For this review, take the finished solid that the model builds, in its own axes (mm). A direction names the side the tool comes from. Round coordinates to 2 decimals unless told otherwise and drop trailing zeros. Write each loop counter-clockwise with the first axis right and the second up, starting at its lowest first coordinate (ties: lowest second). Pieces come first, ordered by that corner, then holes.
from build123d import *

# Parameters (mm, degrees)
SKETCH1_W           = 285.8
SKETCH1_H           = 25.4
BOSS_EXTRUDE1_DEPTH = 25.4
SKETCH2_W           = 23
SKETCH2_H           = 23
CUT_EXTRUDE1_DEPTH  = 450
CUT_EXTRUDE2_DEPTH  = 25.4


with BuildPart() as part:
    # Sketch1 → Boss-Extrude1 (new body)
    with BuildSketch(Plane(origin=(0, 0, 0), x_dir=(1, 0, 0), z_dir=(0, 1, 0))):
        with Locations((142.9, 12.7)):
            Rectangle(SKETCH1_W, SKETCH1_H)
    extrude(amount=BOSS_EXTRUDE1_DEPTH)

    # Sketch2 → Cut-Extrude1 (cut)
    with BuildSketch(Plane(origin=(285.8, 0, 0), x_dir=(0, 0, -1), z_dir=(1, 0, 0))):
        with Locations((12.7, 12.7)):
            Rectangle(SKETCH2_W, SKETCH2_H)
    extrude(amount=-CUT_EXTRUDE1_DEPTH, mode=Mode.SUBTRACT)

    # Sketch3 → Cut-Extrude2 (cut)
    with BuildSketch(Plane(origin=(0, 25.4, 0), x_dir=(1, 0, 0), z_dir=(0, 1, 0))):
        Polygon((0, 0), (25.4, 25.4), (0, 25.4), align=None)
        Polygon((285.8, 0), (260.4, 25.4), (285.8, 25.4), align=None)
    extrude(amount=-CUT_EXTRUDE2_DEPTH, mode=Mode.SUBTRACT)


solid = part.part
(1) We need section C-C, the plane y = 11. Give the boundary of the cut face in (x, z).
Geometry check:
outline: (0, 0) - (1.2, -1.2) - (284.6, -1.2) - (285.8, 0) - close; (24.2, -24.2) - (25.4, -25.4) - (260.4, -25.4) - (261.6, -24.2) - close
(2) We need section A-A, the plane z = -14.75. Give the boundary of the cut face in (x, y).
Geometry check:
outline: (14.75, 0) - (271.05, 0) - (271.05, 1.2) - (14.75, 1.2) - close; (14.75, 24.2) - (271.05, 24.2) - (271.05, 25.4) - (14.75, 25.4) - close
(3) For faces 5 (the face through (145, 13, -1.2)), 6 (the face through (274.1, 0.5, -11.7)), list the 3-axis set-ups (+Z, -Z, +X, -X, +Y, -Y) from which the entire face can be reached by the end or side of a thin tool; tool diameter is ignored.
Geometry check:
face 5: +X, -X
face 6: -Z, +X, +Y, -Y
(4) We need section B-B, the plane x = 202. Give the boundary of the cut face in (y, z), and give its area (3 significant figures).
Geometry check:
outline: (0, -25.4) - (25.4, -25.4) - (25.4, 0) - (0, 0) - close; hole (1.2, -24.2) - (24.2, -24.2) - (24.2, -1.2) - (1.2, -1.2) - close
area: 116 mm2
(5) Mouldability with a two-part tool opening along Y and no side actions: class faces 1 (the face through (141, 0, -13)), 2 (the face through (145, 24.2, -13)), 3 (the face through (145, 13, -24.2)), 4 (the face through (141, 13, -25.4)) as pulls with the +Y half, pulls with the -Y half, needs draft (parallel to the pull), parting line crosses it, or undercut.
Geometry check:
face 1: pulls with the -Y half
face 2: undercut
face 3: undercut
face 4: needs draft
(6) For pin 1 Ø10 at (y, z) = (22, -6) entering from +X, flat-tipped, find the tip position at first contact; note if it passes through.
Geometry check:
pin 1: stops at x = 284.8
(7) For line 1 along Z through (x, y) = (35, 23); line 2 along Y through (x, z) = (31.5, -19.5), list the stretches that pass through material, from the lowest coordinate up.
Geometry check:
line 1: z = -25.4 to -24.2, -1.2 to 0
line 2: y = 0 to 1.2, 24.2 to 25.4
